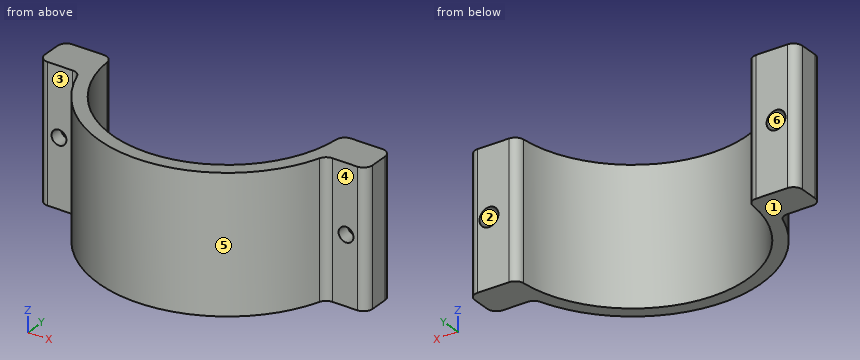
from build123d import *

# Parameters (mm, degrees)
BOSS_EXTRUDE1_DEPTH = 30
SKETCH5_R           = 2.1
CUT_EXTRUDE1_DEPTH  = 5
SKETCH6_R           = 1.65
CUT_EXTRUDE2_DEPTH  = 29.5
FILLET1_R           = 2


with BuildPart() as part:
    # Sketch3 → Boss-Extrude1 (new body)
    with BuildSketch(Plane.XY):
        with BuildLine():
            Line((-25.5, 0), (-36.354158733, 0))
            Line((-36.354158733, 0), (-36.354158733, -8))
            Line((-36.354158733, -8), (-27.354158733, -8))
            ThreePointArc((-27.354158733, -8), (0, -28.5), (27.354158733, -8))
            Line((27.354158733, -8), (36.354158733, -8))
            Line((36.354158733, -8), (36.354158733, 0))
            Line((36.354158733, 0), (25.5, 0))
            ThreePointArc((25.5, 0), (0, -25.5), (-25.5, 0))
        make_face()
    extrude(amount=BOSS_EXTRUDE1_DEPTH)

    # Sketch5 → Cut-Extrude1 (cut)
    with BuildSketch(Plane.XZ):
        with Locations((31.854158733, 15)):
            Circle(SKETCH5_R)
    cut_extrude1 = extrude(amount=CUT_EXTRUDE1_DEPTH, mode=Mode.SUBTRACT)

    # Sketch6 → Cut-Extrude2 (cut, through all)
    with BuildSketch(Plane(origin=(0, 0, 0), x_dir=(1, 0, 0), z_dir=(0, 1, 0))):
        with Locations((31.854158733, -15)):
            Circle(SKETCH6_R)
    cut_extrude2 = extrude(amount=-CUT_EXTRUDE2_DEPTH, mode=Mode.SUBTRACT)

    # Mirror1: Cut-Extrude1, Cut-Extrude2 across plane
    add(cut_extrude1.mirror(Plane(origin=(0, 0, 0), x_dir=(0, 0, 1), z_dir=(1, 0, 0))), mode=Mode.SUBTRACT)
    add(cut_extrude2.mirror(Plane(origin=(0, 0, 0), x_dir=(0, 0, 1), z_dir=(1, 0, 0))), mode=Mode.SUBTRACT)

    # Fillet1
    fillet1_edges = [part.edges().sort_by_distance(p)[0] for p in [
        (-36.354158733, 0, 15),
        (-25.5, 0, 15),
        (25.5, 0, 15),
        (36.354158733, 0, 15),
        (36.354158733, -8, 15),
        (27.354158733, -8, 15),
        (-27.354158733, -8, 15),
        (-36.354158733, -8, 15),
    ]]
    fillet(fillet1_edges, radius=FILLET1_R)


solid = part.part
The listing builds one solid part. Answer for the finished solid, in the listing's coordinates (mm). Face numbers are marked on the shaded views. A direction names the side the tool comes from. Coordinates: 2 decimals unless noted, no trailing zeros. Loops run counter-clockwise (first coordinate to the right, second up) from the corner with the lowest first, then second, coordinate; pieces in that order, holes last.
1) Find the intervals of material crossed by L1, parallel to X at y = -20, z = 1.5; L2, parallel to X at y = -18.25, z = 18; L3, parallel to Y at x = 30, z = 7, in increasing order.
2) Determine the mould class of the marked faces 4, 5 and 6 for opening direction X: pulls with the +X half, pulls with the -X half, needs draft (parallel to the pull), parting line crosses it, or undercut.
3) Find section C-C on y = -4.25. Write down the section's boundary in (x, z).
4) Find section D-D on z = 5.25. Write down the section's boundary in (x, y), then the cut area to 3 significant figures.
5) Flat-ended cylindrical pins translate along their axes: pin 1 Ø3.5 at (x, z) = (-31.5, 15.5) entering from +Y; pin 2 Ø10 at (x, z) = (11, 26.5) entering from -Y; pin 3 Ø8 at (x, z) = (-7, 6.5) entering from -Y; pin 4 Ø4 at (x, z) = (-31.85, 15) entering from +Y. Find the tip coordinate at first contact, or state that the pin passes through.
6) Find section A-A on z = 15. Give the number of separate pieces and of enclosed holes in the cut face, then the cut area to 3 significant figures.
7) Find section B-B on y = -22.5. Write down the section's boundary in (x, z), then the cut area to 3 significant figures.
8) A tool of negligible diameter and unlimited length cuts with its end or side. For the marked faces 1, 2 and 3, from which of +Z, -Z, +X, -X, +Y, -Y can it reach the whole face along a straight path? Write none if from no direction.
Values:
1. L1: x = -20.3 to -15.82, 15.82 to 20.3
1. L2: x = -21.89 to -17.81, 17.81 to 21.89
1. L3: y = -8 to 0
2. face 4: needs draft
2. face 5: parting line crosses it
2. face 6: undercut
3. outline: (-36.35, 0) - (-25.14, 0) - (-25.14, 30) - (-36.35, 30) - close; (25.14, 0) - (36.35, 0) - (36.35, 30) - (25.14, 30) - close; hole circle Ø4.2 at (-31.85, 15); hole circle Ø4.2 at (31.85, 15)
4. outline: (-36.35, -6) arc R2 ccw to (-34.35, -8) - (-28.81, -8) arc R2 cw to (-26.92, -9.34) arc R28.5 ccw to (26.92, -9.34) arc R2 cw to (28.81, -8) - (34.35, -8) arc R2 ccw to (36.35, -6) - (36.35, -2) arc R2 ccw to (34.35, 0) - (27.43, 0) arc R2 ccw to (25.43, -1.85) arc R25.5 cw to (-25.43, -1.85) arc R2 ccw to (-27.43, 0) - (-34.35, 0) arc R2 ccw to (-36.35, -2) - close
4. area: 382 mm2
5. pin 1: stops at y = 0
5. pin 2: stops at y = -27.86
5. pin 3: stops at y = -28.34
5. pin 4: stops at y = -5
6. separate pieces: 3
6. enclosed holes: 0
6. area: 320 mm2
7. outline: (-17.49, 0) - (-12, 0) - (-12, 30) - (-17.49, 30) - close; (12, 0) - (17.49, 0) - (17.49, 30) - (12, 30) - close
7. area: 330 mm2
8. face 1: -Z, +X, -X, +Y, -Y
8. face 2: +Y
8. face 3: +Z, -Z, -X, -Y
